Model file for the job. Use its own axes, mm. A direction names the side the tool comes from. Coordinates: 2 decimals unless noted, no trailing zeros. Write each loop counter-clockwise with the first axis right and the second up, starting at its lowest first coordinate (ties: lowest second). Pieces come first, ordered by that corner, then holes.
Q1. Pin check, flat tips, straight feed: P1, Ø1.9, axis at y = -16.5, z = 3, coming from the +X side; P2, Ø1, axis at x = 61, z = 3.5, coming from the -Y side; P3, Ø3, axis at x = 66.5, z = 2, coming from the -Y side. Stop position of each tip, or through.
Q2. Band-saw the part on C-C, the plane y = 12. Write the cut outline in (x, z).
Q3. Pull direction Y, two halves, no side cores. Call faces 4 (the flat face through (67, -44.45, 3)), 5 (the flat face through (67, 95.25, 3)), 6 (the flat face through (69.85, -69, 3)): released by +Y, released by -Y, zero draft, split by the parting line, or undercut.
Q4. Band-saw the part on A-A, the plane z = 4.75. Write the cut outline in (x, y), plus the area to 3 significant figures.
Q5. Band-saw the part on B-B, the plane x = 5. Write the cut outline in (y, z), plus the area to 3 significant figures.
Q6. Drill centre lines: probe 1 along X at (y, z) = (-14, 2.25); probe 2 along Y at (x, z) = (59, 2.5); probe 3 along Y at (x, z) = (67.5, 6). Where is each one in solid material? Low to high.
Q7. Which spindle directions (+Z, -Z, +X, -X, +Y, -Y) get a long thin tool onto all of the face, cutting with end or side? Do faces 1 (the flat face through (67, 44.45, 3)), 2 (the flat face through (54, -120.65, 3)), 3 (the flat face through (9, -120.65, 3)). Say none if no direction does.
from build123d import *

# Parameters (mm, degrees)
F0_W     = 63.5
F0_H     = 241.3
F1_DEPTH = 6.35
F2_W     = 6.35
F2_H     = 50.8
F3_DEPTH = 6.35
F4_W     = 25.4
F4_H     = 6.35
F5_DEPTH = 6.35


# Not quite as in the source:
# - a pattern or mirror of a feature is missing from the dataset's text; its kind, count and spacing are read off the source's solid


with BuildPart() as f1:
    # F0 (on Top) → F1 (new body)
    with BuildSketch(Plane.XY):
        with Locations((31.75, 0)):
            Rectangle(F0_W, F0_H)
    extrude(amount=F1_DEPTH)

    # F2 (on face) → F3 (join)
    with BuildSketch(Plane.XY.offset(6.35)):
        with Locations((66.675, 69.85)):
            Rectangle(F2_W, F2_H)
    f3 = extrude(amount=-F3_DEPTH)

    # F3_copies: F3 across plane
    add(f3.mirror(Plane(origin=(0, 0, 0), x_dir=(0, 0, -1), z_dir=(0, -1, 0))))

    # F4 (on face) → F5 (join)
    with BuildSketch(Plane.XY.offset(6.35)):
        with Locations((31.75, -123.825)):
            Rectangle(F4_W, F4_H)
    extrude(amount=-F5_DEPTH)


solid = f1.part
Answer sheet:
1. P1: stops at x = 63.5
1. P2: stops at y = -120.65
1. P3: stops at y = -95.25
2. outline: (0, 0) - (63.5, 0) - (63.5, 6.35) - (0, 6.35) - close
3. face 4: undercut
3. face 5: released by +Y
3. face 6: zero draft
4. outline: (0, -120.65) - (19.05, -120.65) - (19.05, -127) - (44.45, -127) - (44.45, -120.65) - (63.5, -120.65) - (63.5, -95.25) - (69.85, -95.25) - (69.85, -44.45) - (63.5, -44.45) - (63.5, 44.45) - (69.85, 44.45) - (69.85, 95.25) - (63.5, 95.25) - (63.5, 120.65) - (0, 120.65) - close
4. area: 16,100 mm2
5. outline: (-120.65, 0) - (120.65, 0) - (120.65, 6.35) - (-120.65, 6.35) - close
5. area: 1,530 mm2
6. probe 1: x = 0 to 63.5
6. probe 2: y = -120.65 to 120.65
6. probe 3: y = -95.25 to -44.45, 44.45 to 95.25
7. face 1: +Z, -Z, +X
7. face 2: +Z, -Z, +X, -Y
7. face 3: +Z, -Z, -X, -Y
